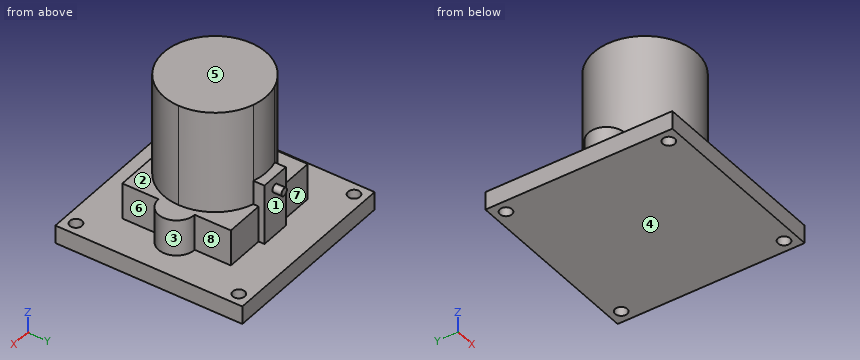
```python
from build123d import *

# Parameters (mm, degrees)
F0_W     = 31
F0_H     = 31
F0_R     = 1
F1_DEPTH = 3
F2_DEPTH = 26
F3_DEPTH = 9
F4_DEPTH = 13
F5_R     = 0.639581
F6_DEPTH = 1.5


with BuildPart() as f1:
    # F0 (on Top) → F1 (new body)
    with BuildSketch(Plane.XY):
        with Locations((0, 2.357912)):
            Rectangle(F0_W, F0_H)
        with Locations((-13.5, -11.142088)):
            Circle(F0_R, mode=Mode.SUBTRACT)
        with Locations((13.5, -11.142088)):
            Circle(F0_R, mode=Mode.SUBTRACT)
        with Locations((-13.5, 15.857912)):
            Circle(F0_R, mode=Mode.SUBTRACT)
        with BuildLine():
            Line((2.5, 11.357912), (9, 11.357912))
            Line((9, 11.357912), (9, 5.357912))
            ThreePointArc((9, 5.357912), (12, 2.357912), (9, -0.642088))
            Line((9, -0.642088), (9, -6.642088))
            Line((9, -6.642088), (-9, -6.642088))
            Line((-9, -6.642088), (-9, -0.642088))
            ThreePointArc((-9, -0.642088), (-12, 2.357912), (-9, 5.357912))
            Line((-9, 5.357912), (-9, 11.357912))
            Line((-9, 11.357912), (-2.5, 11.357912))
            Line((-2.5, 11.357912), (-2.5, 12.327521))
            Line((-2.5, 12.327521), (2.5, 12.327521))
            Line((2.5, 12.327521), (2.5, 11.357912))
        make_face(mode=Mode.SUBTRACT)
        with Locations((13.5, 15.857912)):
            Circle(F0_R, mode=Mode.SUBTRACT)
    extrude(amount=F1_DEPTH)



with BuildPart() as f2:
    # F0 (on Top) → F2 (new body)
    with BuildSketch(Plane.XY):
        with BuildLine():
            ThreePointArc((8.5, 2.357912), (6.837397, 7.407664), (2.5, 10.48195))
            ThreePointArc((2.5, 10.48195), (0, 10.857912), (-2.5, 10.48195))
            ThreePointArc((-2.5, 10.48195), (-5.049752, -4.479485), (8.5, 2.357912))
        make_face()
    extrude(amount=F2_DEPTH)


with BuildPart() as f1_1:
    add(f1.part)

    add(f2.part)  # F3 merges F2
    # F0 (on Top) → F3 (join)
    with BuildSketch(Plane.XY):
        with BuildLine():
            Line((9, 5.357912), (9, 11.357912))
            Line((9, 11.357912), (2.5, 11.357912))
            Line((2.5, 11.357912), (2.5, 10.48195))
            ThreePointArc((2.5, 10.48195), (6.837397, 7.407664), (8.5, 2.357912))
            ThreePointArc((8.5, 2.357912), (-5.049752, -4.479485), (-2.5, 10.48195))
            Line((-2.5, 10.48195), (-2.5, 11.357912))
            Line((-2.5, 11.357912), (-9, 11.357912))
            Line((-9, 11.357912), (-9, 5.357912))
            ThreePointArc((-9, 5.357912), (-12, 2.357912), (-9, -0.642088))
            Line((-9, -0.642088), (-9, -6.642088))
            Line((-9, -6.642088), (9, -6.642088))
            Line((9, -6.642088), (9, -0.642088))
            ThreePointArc((9, -0.642088), (12, 2.357912), (9, 5.357912))
        make_face()
    extrude(amount=F3_DEPTH)

    # F0 (on Top) → F4 (join)
    with BuildSketch(Plane.XY):
        with BuildLine():
            Line((2.5, 10.48195), (2.5, 11.357912))
            Line((2.5, 11.357912), (2.5, 12.327521))
            Line((2.5, 12.327521), (-2.5, 12.327521))
            Line((-2.5, 12.327521), (-2.5, 11.357912))
            Line((-2.5, 11.357912), (-2.5, 10.48195))
            ThreePointArc((-2.5, 10.48195), (0, 10.857912), (2.5, 10.48195))
        make_face()
    extrude(amount=F4_DEPTH)

    # F5 (on face) → F6 (join)
    with BuildSketch(Plane(origin=(0, 12.327521, 0), x_dir=(-1, 0, 0), z_dir=(0, 1, 0))):
        with Locations((0, 11)):
            Circle(F5_R)
    extrude(amount=F6_DEPTH)


with BuildPart() as f7_1:
    # F7: copy of F1
    add(f1_1.part)


solid = f1_1.part
```
Can you work these out from the model? Positions are in its coordinate system, mm. Face numbers are marked on the shaded views. A direction names the side the tool comes from. Round coordinates to 2 decimals unless told otherwise and drop trailing zeros. Loops run counter-clockwise (first coordinate to the right, second up) from the corner with the lowest first, then second, coordinate; pieces in that order, holes last. Notation, with made-up numbers: M 24,-23.75 L 70,-23.75 A30 cw 70,14.25 Z; hole C 36,26.25 d7. An arc over 180 degrees is marked long. Write item = value, one per line. Start each with the question number.
(1) Suppose I cut it at D-D on y = 8. Write out the boundary of the cut face in (x, z).
(2) Suppose I cut it at A-A on x = 0. Write out the boundary of the cut face in (y, z).
(3) Suppose I cut it at C-C on z = 8.5. Write out the boundary of the cut face in (x, y).
(4) I need wall thicknesses on line 1 along Y through (x, z) = (13.5, 2.1); line 2 along Z through (x, y) = (6.5, 16.5); line 3 along Z through (x, y) = (-0.5, 12). Which ranges of each line are inside material? Lowest first, please.
(5) I'm going to push flat-ended pins straight in: P1, Ø1.8, axis at x = 1.5, z = 7, coming from the -Y side; P2, Ø1.5, axis at x = -9.5, y = 3, coming from the +Z side; P3, Ø3, axis at y = -2.5, z = 6.5, coming from the +X side; P4, Ø12, axis at x = -7, y = 8.5, coming from the -Z side. Where does each tip first touch, or does it pass through?
(6) Which directions (+Z, -Z, +X, -X, +Y, -Y) give clear straight access to the entire face, cutting with the end or side of a thin tool? Please do the marked faces 5, 6, 7 and 8.
(7) If we mould it in two halves opening along Z, with no side actions, what happens to the marked faces 1, 2, 3 and 4? For each: released by +Z, released by -Z, zero draft, split by the parting line, or undercut.
(8) Suppose I cut it at B-B on x = -13.5. Write out the boundary of the cut face in (y, z).
Answer block:
q1.outline = M -15.5,0 L 15.5,0 L 15.5,3 L 9,3 L 9,9 L 6.36,9 L 6.36,26 L -6.36,26 L -6.36,9 L -9,9 L -9,3 L -15.5,3 Z
q2.outline = M -13.14,0 L 17.86,0 L 17.86,3 L 12.33,3 L 12.33,10.36 L 13.83,10.36 L 13.83,11.64 L 12.33,11.64 L 12.33,13 L 10.86,13 L 10.86,26 L -6.14,26 L -6.14,9 L -6.64,9 L -6.64,3 L -13.14,3 Z
q3.outline = M -9,-6.64 L 9,-6.64 L 9,-0.64 A3 ccw 9,5.36 L 9,11.36 L 2.5,11.36 L 2.5,12.33 L -2.5,12.33 L -2.5,11.36 L -9,11.36 L -9,5.36 A3 ccw -9,-0.64 Z
q4.line_1 = -13.14 to -12.14, -10.14 to 14.86, 16.86 to 17.86
q4.line_2 = 0 to 3
q4.line_3 = 0 to 13
q5.P1 = -6.64
q5.P2 = 9
q5.P3 = 9
q5.P4 = 0
q6.face_5 = +Z, +X, -X, +Y, -Y
q6.face_6 = +Z, +X, -Y
q6.face_7 = +Z, -X, +Y
q6.face_8 = +Z, +X, +Y
q7.face_1 = undercut
q7.face_2 = released by +Z
q7.face_3 = zero draft
q7.face_4 = released by -Z
q8.outline = M -13.14,0 L -12.14,0 L -12.14,3 L -13.14,3 Z; M -10.14,0 L 14.86,0 L 14.86,3 L -10.14,3 Z; M 16.86,0 L 17.86,0 L 17.86,3 L 16.86,3 Z
